Here's the drawing with two shaded views (mm, measured from the low corner). I have some questions. Round coordinates to 2 decimals unless told otherwise and drop trailing zeros. Loops run counter-clockwise (first coordinate to the right, second up) from the corner with the lowest first, then second, coordinate; pieces in that order, holes last. Notation, with made-up numbers: (29.5, -10.5) -> (66.5, -10.5) arc R25 cw to (66.5, 2.5) -> close; hole circle Ø11 at (80.25, 39). An arc over 180 degrees is marked (long way). Use a Markdown table: item, result.
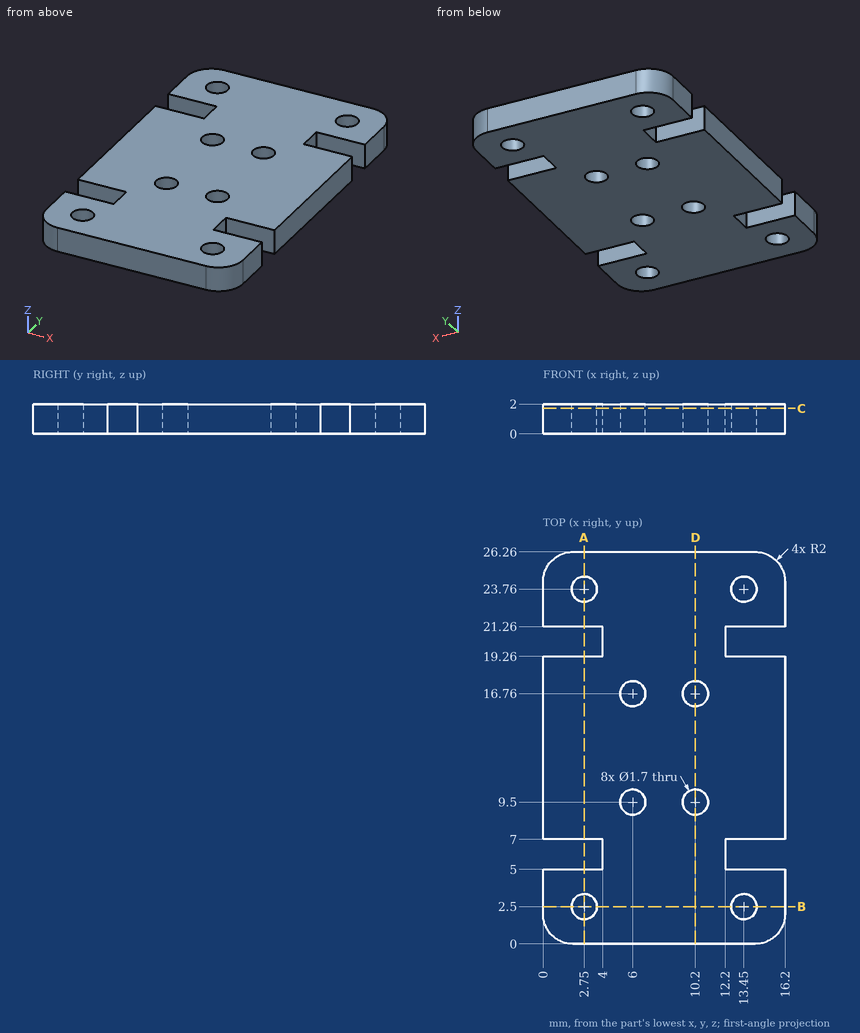
1. Will these pins go through, and if not, where does the flat tip stop? pin 1 Ø1 at (y, z) = (20.5, 1) entering from +X; pin 2 Ø1 at (x, z) = (15, 1) entering from -Y; pin 3 Ø1 at (x, z) = (15, 1) entering from +Y.
Answer sheet:
| item | result |
|---|---|
| pin 1 | stops at x = 12.2 |
| pin 2 | stops at y = 0.02 |
| pin 3 | stops at y = 26.24 |
2. I want a section at C-C (z = 1.7). State how many separate pieces and enclosed holes the cut face has, plus the area to 3 significant figures.
Answer sheet:
| item | result |
|---|---|
| separate pieces | 1 |
| enclosed holes | 8 |
| area | 372 mm² |
3. I want a section at B-B (y = 2.5). Please give me the cut outline in (x, z), plus the area to 3 significant figures.
Answer sheet:
| item | result |
|---|---|
| outline | (0, 0) -> (1.9, 0) -> (1.9, 2) -> (0, 2) -> close; (3.6, 0) -> (12.6, 0) -> (12.6, 2) -> (3.6, 2) -> close; (14.3, 0) -> (16.2, 0) -> (16.2, 2) -> (14.3, 2) -> close |
| area | 25.6 mm² |
4. I want a section at D-D (x = 10.2). Please give me the cut outline in (y, z), plus the area to 3 significant figures.
Answer sheet:
| item | result |
|---|---|
| outline | (0, 0) -> (8.65, 0) -> (8.65, 2) -> (0, 2) -> close; (10.35, 0) -> (15.91, 0) -> (15.91, 2) -> (10.35, 2) -> close; (17.61, 0) -> (26.26, 0) -> (26.26, 2) -> (17.61, 2) -> close |
| area | 45.7 mm² |
5. I want a section at A-A (x = 2.75). Please give me the cut outline in (y, z).
Answer sheet:
| item | result |
|---|---|
| outline | (0, 0) -> (1.65, 0) -> (1.65, 2) -> (0, 2) -> close; (3.35, 0) -> (5, 0) -> (5, 2) -> (3.35, 2) -> close; (7, 0) -> (19.26, 0) -> (19.26, 2) -> (7, 2) -> close; (21.26, 0) -> (22.91, 0) -> (22.91, 2) -> (21.26, 2) -> close; (24.61, 0) -> (26.26, 0) -> (26.26, 2) -> (24.61, 2) -> close |
6. I need wall thicknesses on line 1 (X direction, y = 16.76, z = 0.55); line 2 (Y direction, x = 2.75, z = 1.15); line 3 (Y direction, x = 10.2, z = 1.55). Which ranges of each line are inside material? Lowest first, please.
Answer sheet:
| item | result |
|---|---|
| line 1 | x = 0 to 5.15, 6.85 to 9.35, 11.05 to 16.2 |
| line 2 | y = 0 to 1.65, 3.35 to 5, 7 to 19.26, 21.26 to 22.91, 24.61 to 26.26 |
| line 3 | y = 0 to 8.65, 10.35 to 15.91, 17.61 to 26.26 |
